Autodesk Inventor part; units mm, degrees
ref_plane "YZ Plane" through (0, 0, 0) normal (1, 0, 0) x (0, 1, 0)
ref_plane "XZ Plane" through (0, 0, 0) normal (0, 1, 0) x (-1, 0, 0)
ref_plane "XY Plane" through (0, 0, 0) normal (0, 0, 1) x (1, 0, 0)
sketch "Sketch1" plane through (0, 0, 0) normal (0, 0, 1) x (1, 0, 0)
  line L0 (0, 0) -> (57.3, 0)
  line L1 (57.3, 0) -> (57.3, 57.3)
  line L2 (57.3, 57.3) -> (0, 57.3)
  line L3 (0, 57.3) -> (0, 0)
  line L4 (5.08, 52.22) -> (52.22, 52.22) construction
  line L5 (52.22, 52.22) -> (52.22, 5.08) construction
  line L6 (52.22, 5.08) -> (5.08, 5.08) construction
  line L7 (5.08, 5.08) -> (5.08, 52.22) construction
  line L8 (5.08, 52.22) -> (5.08, 57.3) construction
  line L9 (5.08, 52.22) -> (0, 52.22) construction
  line L10 (52.22, 5.08) -> (52.22, 0) construction
  line L11 (52.22, 5.08) -> (57.3, 5.08) construction
  circle A0 centre (5.08, 52.22) radius 2.55
  circle A1 centre (52.22, 52.22) radius 2.55
  circle A2 centre (5.08, 5.08) radius 2.55
  circle A3 centre (52.22, 5.08) radius 2.55
  line L12 (28.65, 57.3) -> (28.65, 0) construction
  circle A4 centre (28.65, 28.65) radius 19.55
  dimension "d0" = 57.3
  dimension "d1" = 57.3
  dimension "d2" = 47.14
  dimension "d3" = 47.14
  dimension "d4" = 5.1
  dimension "d5" = 5.1
  dimension "d6" = 5.1
  dimension "d7" = 5.1
  dimension "d8" = 39.1
extrude "Extrusion1" add sketch "Sketch1" against normal blind 4 contours L3 L2 L1 L0 | A4
sketch "Sketch2" plane through (0, 0, 0) normal (0, 0, 1) x (1, 0, 0)
  line L0 (0, 57.3) -> (57.3, 57.3) construction
  line L1 (28.65, 57.3) -> (28.65, 0) construction
  line L2 (57.3, 0) -> (0, 0) construction
  circle A0 centre (28.65, 28.65) radius 19.05
  dimension "d11" = 38.1
extrude "Extrusion2" add sketch "Sketch2" along normal blind 1.6
sketch "Sketch3" plane through (28.65, 28.65, 1.6) normal (0, 0, 1) x (1, 0, 0)
  circle A0 centre (0, 0) radius 3.175
  point P0 (-28.65, -28.65)
  dimension "d14" = 6.35
extrude "Extrusion3" add sketch "Sketch3" along normal blind 21
sketch "Sketch4" plane through (28.65, 28.65, 22.6) normal (0, 0, 1) x (1, 0, 0)
  circle A0 centre (0, 0) radius 3.175
  line L0 (-1.7103, 2.675) -> (1.7103, 2.675)
  point P0 (-28.65, -28.65)
  dimension "d17" = 2.675
extrude "Extrusion4" cut sketch "Sketch4" against normal blind 15 contours L0 A0 picked at (-0.3543, 2.7806)
sketch "Sketch5" plane through (0, 0, -4) normal (0, 0, -1) x (-1, 0, 0)
  line L0 (-57.3, 57.3) -> (-57.3, 0)
  line L1 (-57.3, 0) -> (0, 0)
  line L2 (0, 0) -> (0, 57.3)
  line L3 (0, 57.3) -> (-57.3, 57.3)
  circle A0 centre (-5.08, 52.22) radius 2.55
  circle A1 centre (-52.22, 52.22) radius 2.55
  circle A2 centre (-5.08, 5.08) radius 2.55
  circle A3 centre (-52.22, 5.08) radius 2.55
  arc A4 (-52.22, 47.67) -> (-47.67, 52.22) centre (-52.22, 52.22) ccw
  arc A5 (-9.63, 52.22) -> (-5.08, 47.67) centre (-5.08, 52.22) ccw
  arc A6 (-5.08, 9.63) -> (-9.63, 5.08) centre (-5.08, 5.08) ccw
  arc A7 (-47.67, 5.08) -> (-52.22, 9.63) centre (-52.22, 5.08) ccw
  line L4 (0, 57.3) -> (-57.3, 57.3)
  line L5 (-47.67, 55.8) -> (-47.67, 52.22)
  line L6 (-9.63, 55.8) -> (-9.63, 52.22)
  line L7 (-57.3, 0) -> (-57.3, 57.3)
  line L8 (-55.8, 47.67) -> (-52.22, 47.67)
  line L9 (-55.8, 9.63) -> (-52.22, 9.63)
  line L10 (0, 0) -> (-57.3, 0)
  line L11 (-47.67, 1.5) -> (-47.67, 5.08)
  line L12 (-9.63, 1.5) -> (-9.63, 5.08)
  line L13 (0, 57.3) -> (0, 0)
  line L14 (-1.5, 47.67) -> (-5.08, 47.67)
  line L15 (-1.5, 9.63) -> (-5.08, 9.63)
  line L16 (0, 0) -> (0, 57.3)
  line L17 (-57.3, 0) -> (0, 0)
  line L18 (-57.3, 57.3) -> (-57.3, 0)
  arc A8 (-55.8, 47.67) -> (-57.3, 46.17) centre (-55.8, 46.17) ccw
  arc A9 (-46.17, 57.3) -> (-47.67, 55.8) centre (-46.17, 55.8) ccw
  arc A10 (-9.63, 55.8) -> (-11.13, 57.3) centre (-11.13, 55.8) ccw
  arc A11 (0, 46.17) -> (-1.5, 47.67) centre (-1.5, 46.17) ccw
  arc A12 (-1.5, 9.63) -> (0, 11.13) centre (-1.5, 11.13) ccw
  arc A13 (-11.13, 0) -> (-9.63, 1.5) centre (-11.13, 1.5) ccw
  arc A14 (-47.67, 1.5) -> (-46.17, 0) centre (-46.17, 1.5) ccw
  arc A15 (-57.3, 11.13) -> (-55.8, 9.63) centre (-55.8, 11.13) ccw
  dimension "d20" = 2
  dimension "d21" = 2
  dimension "d22" = 2
  dimension "d23" = 2
  dimension "d24" = 3
  dimension "d25" = 3
  dimension "d26" = 3
  dimension "d27" = 3
  dimension "d28" = 3
  dimension "d29" = 3
  dimension "d30" = 3
  dimension "d31" = 3
extrude "Extrusion5" add sketch "Sketch5" along normal blind 4 contours A8 L8 A4 L5 A9 L3 A10 L6 A5 L14 A11 L2 A12 L15 A6 L12 A13 L1 A14 L11 A7 L9 A15 L0
sketch "Sketch6" plane through (0, 0, -8) normal (0, 0, -1) x (-1, 0, 0)
  arc A0 (-52.22, 47.67) -> (-47.67, 52.22) centre (-52.22, 52.22) ccw
  line L0 (-52.22, 47.67) -> (-55.8, 47.67)
  arc A1 (-55.8, 47.67) -> (-57.3, 46.17) centre (-55.8, 46.17) ccw
  line L1 (-57.3, 46.17) -> (-57.3, 11.13)
  arc A2 (-57.3, 11.13) -> (-55.8, 9.63) centre (-55.8, 11.13) ccw
  line L2 (-55.8, 9.63) -> (-52.22, 9.63)
  arc A3 (-47.67, 5.08) -> (-52.22, 9.63) centre (-52.22, 5.08) ccw
  line L3 (-47.67, 5.08) -> (-47.67, 1.5)
  arc A4 (-47.67, 1.5) -> (-46.17, 0) centre (-46.17, 1.5) ccw
  line L4 (-46.17, 0) -> (-11.13, 0)
  arc A5 (-11.13, 0) -> (-9.63, 1.5) centre (-11.13, 1.5) ccw
  line L5 (-9.63, 1.5) -> (-9.63, 5.08)
  arc A6 (-5.08, 9.63) -> (-9.63, 5.08) centre (-5.08, 5.08) ccw
  line L6 (-5.08, 9.63) -> (-1.5, 9.63)
  arc A7 (-1.5, 9.63) -> (0, 11.13) centre (-1.5, 11.13) ccw
  line L7 (0, 11.13) -> (0, 46.17)
  arc A8 (0, 46.17) -> (-1.5, 47.67) centre (-1.5, 46.17) ccw
  line L8 (-1.5, 47.67) -> (-5.08, 47.67)
  arc A9 (-9.63, 52.22) -> (-5.08, 47.67) centre (-5.08, 52.22) ccw
  line L9 (-9.63, 52.22) -> (-9.63, 55.8)
  arc A10 (-9.63, 55.8) -> (-11.13, 57.3) centre (-11.13, 55.8) ccw
  line L10 (-11.13, 57.3) -> (-46.17, 57.3)
  arc A11 (-46.17, 57.3) -> (-47.67, 55.8) centre (-46.17, 55.8) ccw
  line L11 (-47.67, 55.8) -> (-47.67, 52.22)
  line L12 (-55.8, 47.47) -> (-52.22, 47.47)
  arc A12 (-52.22, 47.47) -> (-47.47, 52.22) centre (-52.22, 52.22) ccw
  line L13 (-47.47, 52.22) -> (-47.47, 55.8)
  arc A13 (-46.17, 57.1) -> (-47.47, 55.8) centre (-46.17, 55.8) ccw
  line L14 (-46.17, 57.1) -> (-11.13, 57.1)
  arc A14 (-9.83, 55.8) -> (-11.13, 57.1) centre (-11.13, 55.8) ccw
  line L15 (-9.83, 55.8) -> (-9.83, 52.22)
  arc A15 (-9.83, 52.22) -> (-5.08, 47.47) centre (-5.08, 52.22) ccw
  line L16 (-5.08, 47.47) -> (-1.5, 47.47)
  arc A16 (-0.2, 46.17) -> (-1.5, 47.47) centre (-1.5, 46.17) ccw
  line L17 (-0.2, 46.17) -> (-0.2, 11.13)
  arc A17 (-1.5, 9.83) -> (-0.2, 11.13) centre (-1.5, 11.13) ccw
  line L18 (-1.5, 9.83) -> (-5.08, 9.83)
  arc A18 (-5.08, 9.83) -> (-9.83, 5.08) centre (-5.08, 5.08) ccw
  line L19 (-9.83, 5.08) -> (-9.83, 1.5)
  arc A19 (-11.13, 0.2) -> (-9.83, 1.5) centre (-11.13, 1.5) ccw
  line L20 (-11.13, 0.2) -> (-46.17, 0.2)
  arc A20 (-47.47, 1.5) -> (-46.17, 0.2) centre (-46.17, 1.5) ccw
  line L21 (-47.47, 1.5) -> (-47.47, 5.08)
  arc A21 (-47.47, 5.08) -> (-52.22, 9.83) centre (-52.22, 5.08) ccw
  line L22 (-52.22, 9.83) -> (-55.8, 9.83)
  arc A22 (-57.1, 11.13) -> (-55.8, 9.83) centre (-55.8, 11.13) ccw
  line L23 (-57.1, 11.13) -> (-57.1, 46.17)
  arc A23 (-55.8, 47.47) -> (-57.1, 46.17) centre (-55.8, 46.17) ccw
  point P0 (0, 0)
  dimension "d34" = 0.2
extrude "Extrusion6" add sketch "Sketch6" along normal blind 68 contours L12 A12 L13 A13 L14 A14 L15 A15 L16 A16 L17 A17 L18 A18 L19 A19 L20 A20 L21 A21 L22 A22 L23 A23
sketch "Sketch7" plane through (0, 0, -76) normal (0, 0, -1) x (-1, 0, 0)
  arc A0 (-57.1, 11.13) -> (-55.8, 9.83) centre (-55.8, 11.13) ccw
  line L0 (-57.1, 11.13) -> (-57.1, 46.17)
  arc A1 (-55.8, 47.47) -> (-57.1, 46.17) centre (-55.8, 46.17) ccw
  line L1 (-55.8, 47.47) -> (-52.22, 47.47)
  arc A2 (-52.22, 47.47) -> (-47.47, 52.22) centre (-52.22, 52.22) ccw
  line L2 (-47.47, 52.22) -> (-47.47, 55.8)
  arc A3 (-46.17, 57.1) -> (-47.47, 55.8) centre (-46.17, 55.8) ccw
  line L3 (-46.17, 57.1) -> (-11.13, 57.1)
  arc A4 (-9.83, 55.8) -> (-11.13, 57.1) centre (-11.13, 55.8) ccw
  line L4 (-9.83, 55.8) -> (-9.83, 52.22)
  arc A5 (-9.83, 52.22) -> (-5.08, 47.47) centre (-5.08, 52.22) ccw
  line L5 (-5.08, 47.47) -> (-1.5, 47.47)
  arc A6 (-0.2, 46.17) -> (-1.5, 47.47) centre (-1.5, 46.17) ccw
  line L6 (-0.2, 46.17) -> (-0.2, 11.13)
  arc A7 (-1.5, 9.83) -> (-0.2, 11.13) centre (-1.5, 11.13) ccw
  line L7 (-1.5, 9.83) -> (-5.08, 9.83)
  arc A8 (-5.08, 9.83) -> (-9.83, 5.08) centre (-5.08, 5.08) ccw
  line L8 (-9.83, 5.08) -> (-9.83, 1.5)
  arc A9 (-11.13, 0.2) -> (-9.83, 1.5) centre (-11.13, 1.5) ccw
  line L9 (-11.13, 0.2) -> (-46.17, 0.2)
  arc A10 (-47.47, 1.5) -> (-46.17, 0.2) centre (-46.17, 1.5) ccw
  line L10 (-47.47, 1.5) -> (-47.47, 5.08)
  arc A11 (-47.47, 5.08) -> (-52.22, 9.83) centre (-52.22, 5.08) ccw
  line L11 (-52.22, 9.83) -> (-55.8, 9.83)
  arc A12 (-52.22, 47.67) -> (-47.67, 52.22) centre (-52.22, 52.22) ccw
  line L12 (-52.22, 47.67) -> (-55.8, 47.67)
  arc A13 (-55.8, 47.67) -> (-57.3, 46.17) centre (-55.8, 46.17) ccw
  line L13 (-57.3, 46.17) -> (-57.3, 11.13)
  arc A14 (-57.3, 11.13) -> (-55.8, 9.63) centre (-55.8, 11.13) ccw
  line L14 (-55.8, 9.63) -> (-52.22, 9.63)
  arc A15 (-47.67, 5.08) -> (-52.22, 9.63) centre (-52.22, 5.08) ccw
  line L15 (-47.67, 5.08) -> (-47.67, 1.5)
  arc A16 (-47.67, 1.5) -> (-46.17, 0) centre (-46.17, 1.5) ccw
  line L16 (-46.17, 0) -> (-11.13, 0)
  arc A17 (-11.13, 0) -> (-9.63, 1.5) centre (-11.13, 1.5) ccw
  line L17 (-9.63, 1.5) -> (-9.63, 5.08)
  arc A18 (-5.08, 9.63) -> (-9.63, 5.08) centre (-5.08, 5.08) ccw
  line L18 (-5.08, 9.63) -> (-1.5, 9.63)
  arc A19 (-1.5, 9.63) -> (0, 11.13) centre (-1.5, 11.13) ccw
  line L19 (0, 11.13) -> (0, 46.17)
  arc A20 (0, 46.17) -> (-1.5, 47.67) centre (-1.5, 46.17) ccw
  line L20 (-1.5, 47.67) -> (-5.08, 47.67)
  arc A21 (-9.63, 52.22) -> (-5.08, 47.67) centre (-5.08, 52.22) ccw
  line L21 (-9.63, 52.22) -> (-9.63, 55.8)
  arc A22 (-9.63, 55.8) -> (-11.13, 57.3) centre (-11.13, 55.8) ccw
  line L22 (-11.13, 57.3) -> (-46.17, 57.3)
  arc A23 (-46.17, 57.3) -> (-47.67, 55.8) centre (-46.17, 55.8) ccw
  line L23 (-47.67, 55.8) -> (-47.67, 52.22)
  point P0 (0, 0)
extrude "Extrusion7" add sketch "Sketch7" along normal blind 8 contours L0 A1 L1 A2 L2 A3 L3 A4 L4 A5 L5 A6 L6 A7 L7 A8 L8 A9 L9 A10 L10 A11 L11 A0 | A12 L23 A23 L22 A22 L21 A21 L20 A20 L19 A19 L18 A18 L17 A17 L16 A16 L15 A15 L14 A14 L13 A13 L12
sketch "Sketch8" plane through (0, 0, -84) normal (0, 0, -1) x (-1, 0, 0)
  line L0 (-46.17, 0) -> (-11.13, 0) construction
  line L1 (-28.65, 0) -> (-28.65, 57.1) construction
  line L2 (-46.17, 57.1) -> (-11.13, 57.1) construction
  arc A0 (-30.3603, 31.325) -> (-26.9397, 31.325) centre (-28.65, 28.65) ccw
  circle A1 centre (-28.65, 28.65) radius 3.175
  point P0 (0, 0)
  dimension "d39" = 6.35
extrude "Extrusion8" add sketch "Sketch8" along normal blind 15
sketch "Sketch9" plane through (11.13, 0, -76) normal (0, -1, 0) x (1, 0, 0)
  line L0 (0, -8) -> (35.04, -8)
  line L1 (0, 0) -> (35.04, 0)
  line L2 (13.52, -8) -> (21.52, -8)
  line L3 (21.52, -8) -> (21.52, 0)
  line L4 (21.52, 0) -> (13.52, 0)
  line L5 (13.52, 0) -> (13.52, -8)
  line L6 (14.345, -23) -> (20.695, -23) construction
  line L7 (17.52, -23) -> (17.52, 8.4393) construction
  line L8 (17.52, 0) -> (17.52, -8) construction
  point P0 (-11.13, 76)
  point P1 (13.52, 0)
  point P2 (21.52, -8)
  dimension "d42" = 8
  dimension "d43" = 0
extrude "Extrusion9" add sketch "Sketch9" along normal blind 1
equation "\"d5\" = d4"
equation "\"d6\" = d4"
equation "\"d7\" = d4"
equation "\"d25\" = d24"
equation "\"d26\" = d24"
equation "\"d27\" = d24"
equation "\"d28\" = d24"
equation "\"d29\" = d24"
equation "\"d30\" = d24"
equation "\"d31\" = d24"
properties part number "Nema 23 Dual Shaft 87mm Stepper Motor"
Geometry: final body of the model. Coordinates: model frame, mm. A direction names the side the tool comes from. Round coordinates to 2 decimals unless told otherwise and drop trailing zeros. Loops run counter-clockwise (first coordinate to the right, second up) from the corner with the lowest first, then second, coordinate; pieces in that order, holes last. Notation, with made-up numbers: M 34.25,86 L 92.25,86 A17 cw 92.25,101 Z; hole C -33.75,17.25 d7. An arc over 180 degrees is marked long. One line per question, with ' | ' between items.
(1) Cut plane A-A on z = -2.5. Return the cut outline in (x, y).
Check result:
outline: M 0,0 L 57.3,0 L 57.3,57.3 L 0,57.3 Z; hole C 5.08,5.08 d5.1; hole C 5.08,52.22 d5.1; hole C 52.22,5.08 d5.1; hole C 52.22,52.22 d5.1
(2) Cut plane C-C on z = -15. Return the cut outline in (x, y), plus the area to 3 significant figures.
Check result:
outline: M 0.2,11.13 A1.3 ccw 1.5,9.83 L 5.08,9.83 A4.75 cw 9.83,5.08 L 9.83,1.5 A1.3 ccw 11.13,0.2 L 46.17,0.2 A1.3 ccw 47.47,1.5 L 47.47,5.08 A4.75 cw 52.22,9.83 L 55.8,9.83 A1.3 ccw 57.1,11.13 L 57.1,46.17 A1.3 ccw 55.8,47.47 L 52.22,47.47 A4.75 cw 47.47,52.22 L 47.47,55.8 A1.3 ccw 46.17,57.1 L 11.13,57.1 A1.3 ccw 9.83,55.8 L 9.83,52.22 A4.75 cw 5.08,47.47 L 1.5,47.47 A1.3 ccw 0.2,46.17 Z | area: 2,880 mm2
(3) Cut plane B-B on x = 28.65. Return the cut outline in (y, z) (3 decimals), plus the area to 3 significant figures.
Check result:
outline: M -1,-84 L 25.475,-84 L 25.475,-99 L 31.825,-99 L 31.825,-84 L 57.3,-84 L 57.3,-76 L 57.1,-76 L 57.1,-8 L 57.3,-8 L 57.3,0 L 47.7,0 L 47.7,1.6 L 31.825,1.6 L 31.825,7.6 L 31.325,7.6 L 31.325,22.6 L 25.475,22.6 L 25.475,1.6 L 9.6,1.6 L 9.6,0 L 0,0 L 0,-8 L 0.2,-8 L 0.2,-76 L -1,-76 Z | area: 5,080 mm2
(4) Material intervals for line 1 along Y through (x, z) = (5.08, -2.25); line 2 along X through (y, z) = (52, -1); line 3 along Z through (x, y) = (6.5, 26.5), sorted ascending. Write a range as from..to.
Check result:
line 1: y = 0..2.53, 7.63..49.67, 54.77..57.3 | line 2: x = 0..2.54, 7.62..49.68, 54.76..57.3 | line 3: z = -84..0
(5) Access query for faces 5 (the flat face through (47.47, 54, -42)), 6 (the flat face through (54, 3, -4)), 7 (the flat face through (3, 3, -4)), 8 (the flat face through (0.2, 29, -42)), 9 (the flat face through (54.1, 54.3, -4)). Directions: +Z, -Z, +X, -X, +Y, -Y. A direction counts if a zero-diameter tool reaches every point of the face in a straight line with its end or side. Return the directions, or none.
Check result:
face 5: +X, +Y | face 6: -Z, +X, -Y | face 7: -Z, -X, -Y | face 8: -X, +Y, -Y | face 9: -Z, +X, +Y
(6) Pull-direction query (X, two-part tool) for faces 1 (the cylindrical face through (7.51, 5.85, -1.97)), 2 (the flat face through (54, 9.63, -80)), 3 (the flat face through (47.67, 3, -6)), 4 (the cylindrical face through (54.65, 52.99, -1.97)); classes: +X half, -X half, draft (parallel to the pull), parting line (faces both ways), or undercut.
Check result:
face 1: undercut | face 2: draft | face 3: +X half | face 4: undercut
(7) Cut plane D-D on y = 19.5. Return the cut outline in (x, z), plus the area to 3 significant figures.
Check result:
outline: M 0,-84 L 57.3,-84 L 57.3,-76 L 57.1,-76 L 57.1,-8 L 57.3,-8 L 57.3,0 L 45.36,0 L 45.36,1.6 L 11.94,1.6 L 11.94,0 L 0,0 L 0,-8 L 0.2,-8 L 0.2,-76 L 0,-76 Z | area: 4,840 mm2
(8) Contact query for flat-ended pins moving along their axis: P1, Ø10.5, axis at x = 21.5, z = -43, coming from the -Y side; P2, Ø4, axis at x = 54.5, z = -5, coming from the -Y side; P3, Ø0.5, axis at y = -0.5, z = -78, coming from the +X side. Output: stop coordinate, or through.
Check result:
P1: stops at y = 0.2 | P2: stops at y = 0 | P3: stops at x = 32.65
